from build123d import *

# Parameters (mm, degrees)
ESQUISSE1_W             = 31
ESQUISSE1_H             = 23
BOSS_EXTRU_1_DEPTH      = 5
ESQUISSE2_W             = 25
ESQUISSE2_H             = 17
ENL_V_MAT_EXTRU_1_DEPTH = 3
ESQUISSE4_W             = 6
ESQUISSE4_H             = 6
BOSS_EXTRU_3_DEPTH      = 8
CHANFREIN2_SIZE         = 1
CONG_2_R                = 1
ESQUISSE3_R             = 1.5
ENL_V_MAT_EXTRU_2_DEPTH = 3
ESQUISSE5_R             = 1.5
ENL_V_MAT_EXTRU_3_DEPTH = 9


with BuildPart() as part:
    # Esquisse1 → Boss.-Extru.1 (new body)
    with BuildSketch(Plane.XY):
        with Locations((-15.5, 11.5)):
            Rectangle(ESQUISSE1_W, ESQUISSE1_H)
    extrude(amount=BOSS_EXTRU_1_DEPTH)

    # Esquisse2 → Enlèv. mat.-Extru.1 (cut)
    with BuildSketch(Plane.XY.offset(5)):
        with Locations((-15.5, 11.5)):
            Rectangle(ESQUISSE2_W, ESQUISSE2_H)
    extrude(amount=-ENL_V_MAT_EXTRU_1_DEPTH, mode=Mode.SUBTRACT)

    # Esquisse4 → Boss.-Extru.3 (add)
    with BuildSketch(Plane.XY.offset(5)):
        with Locations((-34, 12)):
            Rectangle(ESQUISSE4_W, ESQUISSE4_H)
        with Locations((3, 12)):
            Rectangle(ESQUISSE4_W, ESQUISSE4_H)
    extrude(amount=-BOSS_EXTRU_3_DEPTH)

    # Chanfrein2
    chanfrein2_edges = [part.edges().sort_by_distance(p)[0] for p in [
        (-15.5, 3, 5),
    ]]
    chamfer(chanfrein2_edges, length=CHANFREIN2_SIZE)

    # Congé2
    cong_2_edges = [part.edges().sort_by_distance(p)[0] for p in [
        (-37, 15, 1),
        (6, 15, 1),
        (6, 9, 1),
        (-37, 9, 1),
    ]]
    fillet(cong_2_edges, radius=CONG_2_R)

    # Esquisse3 → Enlèv. mat.-Extru.2 (cut)
    with BuildSketch(Plane.XY.offset(2)):
        with Locations((-26, 18)):
            Circle(ESQUISSE3_R)
        with Locations((-5, 18)):
            Circle(ESQUISSE3_R)
    extrude(amount=-ENL_V_MAT_EXTRU_2_DEPTH, mode=Mode.SUBTRACT)

    # Esquisse5 → Enlèv. mat.-Extru.3 (cut, through all)
    with BuildSketch(Plane.XY.offset(5)):
        with Locations((-34, 12)):
            Circle(ESQUISSE5_R)
        with Locations((3, 12)):
            Circle(ESQUISSE5_R)
    extrude(amount=-ENL_V_MAT_EXTRU_3_DEPTH, mode=Mode.SUBTRACT)


solid = part.part
Here's how the part is built. I have some questions about the finished solid (model axes, mm). A direction names the side the tool comes from. Round coordinates to 2 decimals unless told otherwise and drop trailing zeros. Loops run counter-clockwise (first coordinate to the right, second up) from the corner with the lowest first, then second, coordinate; pieces in that order, holes last.
1. If we section it at B-B on x = -5: Write out the boundary of the cut face in (y, z).
Answer list:
outline: (0, 0) - (16.5, 0) - (16.5, 2) - (3, 2) - (3, 4) - (2, 5) - (0, 5) - close; (19.5, 0) - (23, 0) - (23, 5) - (20, 5) - (20, 2) - (19.5, 2) - close
2. If we section it at C-C on y = 18.5: Write out the boundary of the cut face in (x, z).
Answer list:
outline: (-31, 0) - (-27.41, 0) - (-27.41, 2) - (-28, 2) - (-28, 5) - (-31, 5) - close; (-24.59, 0) - (-6.41, 0) - (-6.41, 2) - (-24.59, 2) - close; (-3.59, 0) - (0, 0) - (0, 5) - (-3, 5) - (-3, 2) - (-3.59, 2) - close
3. If we section it at D-D on x = -34: Write out the boundary of the cut face in (y, z), plus the area to 3 significant figures.
Answer list:
outline: (9, -3) - (10.5, -3) - (10.5, 5) - (9, 5) - close; (13.5, -3) - (15, -3) - (15, 5) - (13.5, 5) - close
area: 24.0 mm2
4. If we section it at A-A on z = -2.5: Write out the boundary of the cut face in (x, y).
Answer list:
outline: (-37, 10) arc R1 ccw to (-36, 9) - (-31, 9) - (-31, 15) - (-36, 15) arc R1 ccw to (-37, 14) - close; (0, 9) - (5, 9) arc R1 ccw to (6, 10) - (6, 14) arc R1 ccw to (5, 15) - (0, 15) - close; hole circle Ø3 at (-34, 12); hole circle Ø3 at (3, 12)
5. For P1, Ø1, axis at x = -11.5, y = 7.5, coming from the +Z side; P2, Ø2.5, axis at y = 19.5, z = 3, coming from the +X side; P3, Ø2.5, axis at x = -26, y = 18, coming from the +Z side (3 decimals); P4, Ø4, axis at x = 3.5, z = 1, coming from the -Y side, each with a flat end and sliding along its axis, tell me the tip position at first contact or that it passes through.
Answer list:
P1: stops at z = 2
P2: stops at x = 0
P3: passes through
P4: stops at y = 9
6. We'd pull the mould along X, two halves only. Please class faces 6 (the face through (-31, 19, 2)), 7 (the face through (0, 4, 2)), 8 (the face through (-3, 11, 4)): +X half, -X half, draft (parallel to the pull), parting line (faces both ways), or undercut.
Answer list:
face 6: -X half
face 7: +X half
face 8: undercut
7. If I drill on line 1 along Y through (x, z) = (3, 0); line 2 along Y through (x, z) = (-5, 0.5); line 3 along X through (y, z) = (11.5, 1.5), over which ranges is the centre line in solid material (lowest first)?
Answer list:
line 1: y = 9 to 10.5, 13.5 to 15
line 2: y = 0 to 16.5, 19.5 to 23
line 3: x = -37 to -35.41, -32.59 to 1.59, 4.41 to 6
8. Which directions (+Z, -Z, +X, -X, +Y, -Y) give clear straight access to the entire face, cutting with the end or side of a thin tool? Please do faces 1 (the face through (-34, 15, 1)), 2 (the face through (-32.7, 10.7, -3)), 3 (the face through (-31, 12, -1)), 4 (the face through (-16, 12, 2)), 5 (the face through (-34, 9, 1)).
Answer list:
face 1: +Z, -Z, -X, +Y
face 2: -Z, +X, -X, +Y, -Y
face 3: -Z, +Y, -Y
face 4: +Z
face 5: +Z, -Z, -X, -Y
